The model under review builds one solid part; all positions refer to its coordinate system, in mm. A direction names the side the tool comes from. Round coordinates to 2 decimals unless told otherwise and drop trailing zeros. Order: outer loops, then holes, each group sorted by start corner. A loop starts at its lowest first (then second) coordinate and runs counter-clockwise, first axis right, second up. Notation, with made-up numbers: (65.25, 56) -> (116.25, 56) arc R37 cw to (116.25, 95) -> close; hole circle Ø11 at (-15, 85.5). An arc over 180 degrees is marked (long way). Use a Markdown table: item, result. Add a question column.
```python
from build123d import *

# Parameters (mm, degrees)
SKETCH1_W            = 35
SKETCH1_H            = 30
BOSS_EXTRUDE1_DEPTH  = 3
SKETCH2_W            = 29
SKETCH2_H            = 24
CUT_EXTRUDE1_DEPTH   = 2
SKETCH5_W            = 4.266255033
SKETCH5_H            = 4
SKETCH5_W_2          = 4
BOSS_EXTRUDE2_DEPTH  = 2
M3_CLEARANCE_HOLE1_D = 3.6
FILLET1_R            = 3
FILLET2_R            = 1


with BuildPart() as part:
    # Sketch1 → Boss-Extrude1 (new body)
    with BuildSketch(Plane(origin=(0, 0, 0), x_dir=(1, 0, 0), z_dir=(0, 1, 0))):
        Rectangle(SKETCH1_W, SKETCH1_H)
    extrude(amount=BOSS_EXTRUDE1_DEPTH)

    # Sketch2 → Cut-Extrude1 (cut)
    with BuildSketch(Plane(origin=(0, 3, 0), x_dir=(1, 0, 0), z_dir=(0, 1, 0))):
        Rectangle(SKETCH2_W, SKETCH2_H)
    extrude(amount=-CUT_EXTRUDE1_DEPTH, mode=Mode.SUBTRACT)

    # Sketch5 → Boss-Extrude2 (add)
    with BuildSketch(Plane(origin=(0, 1, 0), x_dir=(1, 0, 0), z_dir=(0, 1, 0))):
        with Locations((-12.366872483, 10)):
            Rectangle(SKETCH5_W, SKETCH5_H)
        with Locations((12.5, 10)):
            Rectangle(SKETCH5_W_2, SKETCH5_H)
        with Locations((12.5, -10)):
            Rectangle(SKETCH5_W_2, SKETCH5_H)
        with Locations((-12.5, -10)):
            Rectangle(SKETCH5_W_2, SKETCH5_H)
    extrude(amount=BOSS_EXTRUDE2_DEPTH)

    # M3 Clearance Hole1 (through all)
    with Locations(Plane(origin=(0, 3, 0), x_dir=(1, 0, 0), z_dir=(0, 1, 0))):
        with Locations((0, 0), (13, 11), (-13, -11), (-13, 11), (13, -11)):
            Hole(M3_CLEARANCE_HOLE1_D / 2)

    # Fillet1
    fillet1_edges = [part.edges().sort_by_distance(p)[0] for p in [
        (17.5, 1.5, 15),
        (-17.5, 1.5, 15),
        (-17.5, 1.5, -15),
        (17.5, 1.5, -15),
    ]]
    fillet(fillet1_edges, radius=FILLET1_R)

    # Fillet2
    fillet2_edges = [part.edges().sort_by_distance(p)[0] for p in [
        (-10.233744967, 2, -8),
        (10.5, 2, -8),
        (10.5, 2, 8),
        (-10.5, 2, 8),
    ]]
    fillet(fillet2_edges, radius=FILLET2_R)


solid = part.part
```
Q1. Mouldability with a two-part tool opening along X and no side actions: class faces 3 (the flat face through (-17.5, 1, 0)), 4 (the cylindrical face through (-10.53, 2.01, -8.29)), 5 (the flat face through (0, 1, 15)) as pulls with the +X half, pulls with the -X half, needs draft (parallel to the pull), parting line crosses it, or undercut.
Q2. Add section A-A (x = 0). Write out the cut boundary in (y, z).
Q3. Add section B-B (z = 11). Write out the cut boundary in (x, y).
Q4. Machinability: for faces 1 (the flat face through (-10.234, 2, -10)), 2 (the cylindrical face through (16.6, 1.52, 14.14)), which of the approach directions +Z, -Z, +X, -X, +Y, -Y give a long, thin tool a straight path to every point of the face, cutting with its end or side? Answer none if there is none.
Q5. Add section D-D (z = 0). Write out the cut boundary in (x, y), then the cut area to 3 significant figures.
Q6. Add section C-C (x = 13). Write out the cut boundary in (y, z), then the cut area to 3 significant figures.
Q7. Wall thickness on line 1 (X direction, y = 1.65, z = 11); line 2 (X direction, y = 1.9, z = -11); line 3 (Z direction, x = -13, y = 1.95): over which ranges is each line inside the solid? List them lowest first. Write a range as [from, to].
Q8. Insertion check: pin 1 (7 mm diameter, centred on x = -3.5, z = -1, fed in from +Y); pin 2 (2 mm diameter, centred on x = -13, z = 11, fed in from +Y). Each pin has a flat end and moves straight along its axis. Give the tip position at first contact, or say it passes through.
Report:
| question | item | result |
|---|---|---|
| 1 | face 3 | pulls with the -X half |
| 1 | face 4 | undercut |
| 1 | face 5 | needs draft |
| 2 | outline | (0, -15) -> (3, -15) -> (3, -12) -> (1, -12) -> (1, -1.8) -> (0, -1.8) -> close; (0, 1.8) -> (1, 1.8) -> (1, 12) -> (3, 12) -> (3, 15) -> (0, 15) -> close |
| 3 | outline | (-17.5, 0) -> (-14.8, 0) -> (-14.8, 3) -> (-17.5, 3) -> close; (-11.2, 0) -> (11.2, 0) -> (11.2, 3) -> (10.5, 3) -> (10.5, 1) -> (-10.5, 1) -> (-10.5, 3) -> (-11.2, 3) -> close; (14.8, 0) -> (17.5, 0) -> (17.5, 3) -> (14.8, 3) -> close |
| 4 | face 1 | +Y |
| 4 | face 2 | +Z, +X, +Y, -Y |
| 5 | outline | (-17.5, 0) -> (-1.8, 0) -> (-1.8, 1) -> (-14.5, 1) -> (-14.5, 3) -> (-17.5, 3) -> close; (1.8, 0) -> (17.5, 0) -> (17.5, 3) -> (14.5, 3) -> (14.5, 1) -> (1.8, 1) -> close |
| 5 | area | 43.4 mm² |
| 6 | outline | (0, -15) -> (3, -15) -> (3, -12.8) -> (0, -12.8) -> close; (0, -9.2) -> (3, -9.2) -> (3, -8) -> (1, -8) -> (1, 8) -> (3, 8) -> (3, 9.2) -> (0, 9.2) -> close; (0, 12.8) -> (3, 12.8) -> (3, 15) -> (0, 15) -> close |
| 6 | area | 36.4 mm² |
| 7 | line 1 | x = [-17.5, -14.8], [-11.2, -10.5], [10.5, 11.2], [14.8, 17.5] |
| 7 | line 2 | x = [-17.5, -14.8], [-11.2, -10.23], [10.5, 11.2], [14.8, 17.5] |
| 7 | line 3 | z = [-15, -12.8], [-9.2, -8], [8, 9.2], [12.8, 15] |
| 8 | pin 1 | stops at y = 1 |
| 8 | pin 2 | passes through |
